```python
from build123d import *

# Parameters (mm, degrees)
SKETCH1_W           = 96.5
SKETCH1_H           = 110
BOSS_EXTRUDE1_DEPTH = 4.5
SKETCH2_R           = 4
BOSS_EXTRUDE2_DEPTH = 4
SKETCH3_R           = 2
BOSS_EXTRUDE3_DEPTH = 14.4
SKETCH4_W           = 20
SKETCH4_H           = 37.6
BOSS_EXTRUDE4_DEPTH = 1.75
BOSS_EXTRUDE5_DEPTH = 11.5
BOSS_EXTRUDE6_DEPTH = 5.3
CHAMFER2_SIZE       = 1
CUT_EXTRUDE6_DEPTH  = 115.67545509
CHAMFER3_SIZE       = 1
SKETCH2_4_R         = 4
BOSS_EXTRUDE8_DEPTH = 4
CUT_EXTRUDE10_DEPTH = 148.036084007
FILLET1_R           = 10
SKETCH21_R          = 2
CUT_EXTRUDE11_DEPTH = 148.036084007
CHAMFER4_SIZE       = 1
SKETCH22_R          = 2
CUT_EXTRUDE12_DEPTH = 147.698363999
FILLET2_R           = 25


with BuildPart() as part:
    # Sketch1 → Boss-Extrude1 (new body)
    with BuildSketch(Plane(origin=(0, 0, 0), x_dir=(1, 0, 0), z_dir=(0, 1, 0))):
        with Locations((48.25, -55)):
            Rectangle(SKETCH1_W, SKETCH1_H)
    extrude(amount=BOSS_EXTRUDE1_DEPTH)

    # Sketch2 → Boss-Extrude2 (add)
    with BuildSketch(Plane(origin=(0, 4.5, 0), x_dir=(1, 0, 0), z_dir=(0, 1, 0))):
        with Locations(Location((25, -100, 0), (0, 0, 270))):
            Circle(SKETCH2_R)
        with Locations(Location((71.5, -100, 0), (0, 0, 270))):
            Circle(SKETCH2_R)
    extrude(amount=BOSS_EXTRUDE2_DEPTH)

    # Sketch3 → Boss-Extrude3 (add)
    with BuildSketch(Plane(origin=(0, 4.5, 0), x_dir=(1, 0, 0), z_dir=(0, 1, 0))):
        with Locations(Location((48.25, -16.9, 0), (0, 0, 270))):
            Circle(SKETCH3_R)
    extrude(amount=BOSS_EXTRUDE3_DEPTH)

    # Sketch4 → Boss-Extrude4 (add)
    with BuildSketch(Plane(origin=(0, 4.5, 0), x_dir=(1, 0, 0), z_dir=(0, 1, 0))):
        with Locations((48.25, -40.2)):
            Rectangle(SKETCH4_W, SKETCH4_H)
    extrude(amount=BOSS_EXTRUDE4_DEPTH)

    # Sketch4<3> → Boss-Extrude5 (add)
    with BuildSketch(Plane(origin=(0, 4.5, 0), x_dir=(1, 0, 0), z_dir=(0, 1, 0))):
        Polygon((58.25, -59), (58.25, -95), (38.25, -95), (38.25, -59), (48.25, -59), align=None)
    extrude(amount=BOSS_EXTRUDE5_DEPTH)

    # Sketch4<5> → Boss-Extrude6 (add)
    with BuildSketch(Plane(origin=(0, 4.5, 0), x_dir=(1, 0, 0), z_dir=(0, 1, 0))):
        with BuildLine():
            Line((49.25, -12.4), (47.25, -12.4))
            ThreePointArc((47.25, -12.4), (44.421572875, -13.571572875), (43.25, -16.4))
            Line((43.25, -16.4), (43.25, -21.4))
            Line((43.25, -21.4), (53.25, -21.4))
            Line((53.25, -21.4), (53.25, -16.4))
            ThreePointArc((53.25, -16.4), (52.078427125, -13.571572875), (49.25, -12.4))
        make_face()
    extrude(amount=BOSS_EXTRUDE6_DEPTH)

    # Chamfer2
    chamfer2_edges = [part.edges().sort_by_distance(p)[0] for p in [
        (48.25, 18.9, 14.9),
    ]]
    chamfer(chamfer2_edges, length=CHAMFER2_SIZE)

    # Sketch9 → Cut-Extrude6 (cut, through all)
    with BuildSketch(Plane(origin=(0, 0, 59), x_dir=(-1, 0, 0), z_dir=(0, 0, -1))):
        with BuildLine():
            ThreePointArc((-55.849342077, 16), (-55.970490222, 11.403805654), (-53.541502622, 7.5))
            Line((-53.541502622, 7.5), (-42.958497378, 7.5))
            ThreePointArc((-42.958497378, 7.5), (-40.958497378, 10.208497378), (-40.25, 13.5))
            ThreePointArc((-40.25, 13.5), (-40.350799515, 14.765950905), (-40.650657923, 16))
            Line((-40.650657923, 16), (-55.849342077, 16))
        make_face()
    extrude(amount=-CUT_EXTRUDE6_DEPTH, mode=Mode.SUBTRACT)

    # Chamfer3
    chamfer3_edges = [part.edges().sort_by_distance(p)[0] for p in [
        (25, 8.5, 96),
        (71.5, 8.5, 96),
    ]]
    chamfer(chamfer3_edges, length=CHAMFER3_SIZE)

    # Sketch2<4> → Boss-Extrude8 (add)
    with BuildSketch(Plane(origin=(0, 4.5, 0), x_dir=(1, 0, 0), z_dir=(0, 1, 0))):
        with Locations(Location((11, -90, 0), (0, 0, 270))):
            Circle(SKETCH2_4_R)
        with Locations(Location((85.5, -90, 0), (0, 0, 270))):
            Circle(SKETCH2_4_R)
    extrude(amount=BOSS_EXTRUDE8_DEPTH)

    # Sketch20 → Cut-Extrude10 (cut, through all)
    with BuildSketch(Plane(origin=(0, 4.5, 0), x_dir=(1, 0, 0), z_dir=(0, 1, 0))):
        with BuildLine():
            Line((0, 0), (96.5, 0))
            Line((96.5, 0), (96.5, -54.687652439))
            ThreePointArc((96.5, -54.687652439), (77.742842614, -48.529130099), (58.25, -45.400642056))
            Line((58.25, -45.400642056), (58.25, -21.4))
            Line((58.25, -21.4), (53.25, -21.4))
            Line((53.25, -21.4), (53.25, -16.4))
            ThreePointArc((53.25, -16.4), (52.078427125, -13.571572875), (49.25, -12.4))
            Line((49.25, -12.4), (47.25, -12.4))
            ThreePointArc((47.25, -12.4), (44.421572875, -13.571572875), (43.25, -16.4))
            Line((43.25, -16.4), (43.25, -21.4))
            Line((43.25, -21.4), (38.25, -21.4))
            Line((38.25, -21.4), (38.25, -45.400642056))
            ThreePointArc((38.25, -45.400642056), (18.757157386, -48.529130099), (0, -54.687652439))
            Line((0, -54.687652439), (0, 0))
        make_face()
    extrude(amount=-CUT_EXTRUDE10_DEPTH, mode=Mode.SUBTRACT)

    # Fillet1
    fillet1_edges = [part.edges().sort_by_distance(p)[0] for p in [
        (58.25, 2.25, 45.400642056),
        (38.25, 2.25, 45.400642056),
    ]]
    fillet(fillet1_edges, radius=FILLET1_R)

    # Sketch21 → Cut-Extrude11 (cut, through all)
    with BuildSketch(Plane(origin=(0, 4.5, 0), x_dir=(1, 0, 0), z_dir=(0, 1, 0))):
        with Locations(Location((21.588470277, -60.190333609, 0), (0, 0, 270))):
            Circle(SKETCH21_R)
        with Locations(Location((74.911529723, -60.190333609, 0), (0, 0, 270))):
            Circle(SKETCH21_R)
    extrude(amount=-CUT_EXTRUDE11_DEPTH, mode=Mode.SUBTRACT)

    # Chamfer4
    chamfer4_edges = [part.edges().sort_by_distance(p)[0] for p in [
        (11, 8.5, 86),
        (85.5, 8.5, 86),
    ]]
    chamfer(chamfer4_edges, length=CHAMFER4_SIZE)

    # Sketch22 → Cut-Extrude12 (cut, through all)
    with BuildSketch(Plane(origin=(0, 8.5, 0), x_dir=(1, 0, 0), z_dir=(0, 1, 0))):
        with Locations(Location((11, -90, 0), (0, 0, 270))):
            Circle(SKETCH22_R)
        with Locations(Location((85.5, -90, 0), (0, 0, 270))):
            Circle(SKETCH22_R)
    extrude(amount=-CUT_EXTRUDE12_DEPTH, mode=Mode.SUBTRACT)

    # Fillet2
    fillet2_edges = [part.edges().sort_by_distance(p)[0] for p in [
        (96.5, 2.25, 110),
        (0, 2.25, 110),
    ]]
    fillet(fillet2_edges, radius=FILLET2_R)


solid = part.part
```
Verification items for the finished model (mm, model axes). A direction names the side the tool comes from. Give positions to 0.01 mm unless a question says otherwise; leave off trailing zeros. Order: outer loops, then holes, each group sorted by start corner. A loop starts at its lowest first (then second) coordinate and runs counter-clockwise, first axis right, second up. Notation, with made-up numbers: (11, 81) -> (54, 81) arc R19 cw to (54, 109) -> close; hole circle Ø3 at (78, 57). An arc over 180 degrees is marked (long way). Use a Markdown table: item, result.
1) Section check D-D, the plane z = 32. Record the boundary of the cut face in (x, y).
Results:
| item | result |
|---|---|
| outline | (38.25, 0) -> (58.25, 0) -> (58.25, 6.25) -> (38.25, 6.25) -> close |
2) Depth check by flat-ended pin: pin 1 Ø6 at (x, y) = (59, 12.5) entering from +Z; pin 2 Ø4 at (y, z) = (5.5, 18.5) entering from -X; pin 3 Ø3 at (x, z) = (11, 89) entering from +Y; pin 4 Ø3 at (x, y) = (78, 9) entering from -Z. Enter the tip coordinate at first touch or a pass-through.
Results:
| item | result |
|---|---|
| pin 1 | z = 95 |
| pin 2 | x = 43.25 |
| pin 3 | y = 8.5 |
| pin 4 | through |
3) Section check C-C, the plane y = 11.75. Record the boundary of the cut face in (x, z), then the cut area to 3 significant figures.
Results:
| item | result |
|---|---|
| outline | (38.25, 59) -> (40.44, 59) -> (40.44, 95) -> (38.25, 95) -> close; circle Ø4 at (48.25, 16.9); (56.06, 59) -> (58.25, 59) -> (58.25, 95) -> (56.06, 95) -> close |
| area | 171 mm² |
4) Material ranges on probe 1 along Y at (x, z) = (58, 105); probe 2 along X at (y, z) = (5.5, 41.5); probe 3 along X at (y, z) = (2.25, 16), recorded low to high.
Results:
| item | result |
|---|---|
| probe 1 | 0 to 4.5 |
| probe 2 | 38.25 to 58.25 |
| probe 3 | 43.27 to 53.23 |
5) Tool access check on faces 1 (the flat face through (88, 8.5, 90)), 2 (the flat face through (43.25, 5, 19)), 3 (the cylindrical face through (55.99, 11.47, 76.75)), 4 (the cylindrical face through (88.982, 2.282, 102.871)), 5 (the flat face through (49, 9.8, 19)). Record the directions out of +Z, -Z, +X, -X, +Y, -Y that give a thin tool (end or side, any length) a straight path to the whole face; none if there is none.
Results:
| item | result |
|---|---|
| face 1 | +Z, -Z, +X, +Y |
| face 2 | -Z, -X, +Y, -Y |
| face 3 | +Z, -Z |
| face 4 | +Z, +X, +Y, -Y |
| face 5 | +Y |
6) Section check A-A, the plane x = 85.5. Record the boundary of the cut face in (y, z), then the cut area to 3 significant figures.
Results:
| item | result |
|---|---|
| outline | (0, 50.68) -> (4.5, 50.68) -> (4.5, 86) -> (7.5, 86) -> (8.5, 87) -> (8.5, 88) -> (0, 88) -> close; (0, 92) -> (8.5, 92) -> (8.5, 93) -> (7.5, 94) -> (4.5, 94) -> (4.5, 105.71) -> (0, 105.71) -> close |
| area | 245 mm² |
7) Mould release check, pull along X, two halves, no side actions. Record for faces 6 (the flat face through (57, 16, 77)), 7 (the flat face through (37, 4.5, 81)), 8 (the cylindrical face through (44.453, 4.969, 13.541)): pulls with the +X half, pulls with the -X half, needs draft (parallel to the pull), parting line crosses it, or undercut.
Results:
| item | result |
|---|---|
| face 6 | needs draft |
| face 7 | undercut |
| face 8 | pulls with the -X half |
8) Section check B-B, the plane z = 67. Record the boundary of the cut face in (x, y), then the cut area to 3 significant figures.
Results:
| item | result |
|---|---|
| outline | (0, 0) -> (96.5, 0) -> (96.5, 4.5) -> (58.25, 4.5) -> (58.25, 16) -> (55.85, 16) arc R8 cw to (53.54, 7.5) -> (42.96, 7.5) arc R8 cw to (40.65, 16) -> (38.25, 16) -> (38.25, 4.5) -> (0, 4.5) -> close |
| area | 539 mm² |
